Geometry: final body of the model. Coordinates: model frame, mm. Face numbers are marked on the shaded views. A direction names the side the tool comes from. Give positions to 0.01 mm unless a question says otherwise; leave off trailing zeros. Write each loop counter-clockwise with the first axis right and the second up, starting at its lowest first coordinate (ties: lowest second). Pieces come first, ordered by that corner, then holes.
Q1. Section D-D (z = 20). Return the cut outline in (x, y), plus the area to 3 significant figures.
Q2. Pin query (flat end, axial travel): pin 1 Ø1 at (x, y) = (54.5, 40.5) entering from +Z; pin 2 Ø1.9 at (x, y) = (38.5, 3.5) entering from +Z; pin 3 Ø1 at (x, y) = (32, 3.5) entering from +Z. Return the tip coordinate at first contact, or that it passes through.
Q3. Section A-A (z = 15). Return the cut outline in (x, y).
Q4. Reachability of the marked faces 1 and 2 from +Z, -Z, +X, -X, +Y, -Y: full face, straight path, thin tool, end or side. Return the list, or none.
Q5. Mould query, pull axis X, two halves, no side actions, for the marked faces 3, 4 and 5. Classes: +X half, -X half, draft (parallel to the pull), parting line (faces both ways), or undercut.
Q6. Section C-C (x = 35.5). Return the cut outline in (y, z), plus the area to 3 significant figures.
Q7. Section B-B (y = 35). Return the cut outline in (x, z).
Q8. Line query: line 1 (Y direction, x = 32, z = 23); line 2 (Y direction, x = 27, z = 22). Output: solid intervals per line, ascending.
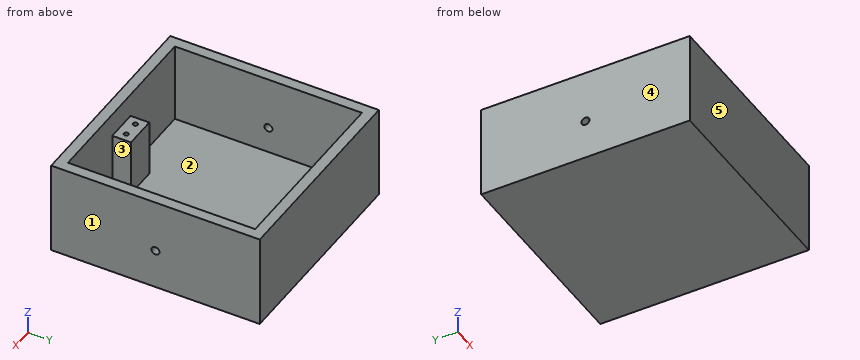
from build123d import *

# Parameters (mm, degrees)
F0_W      = 78
F0_H      = 78
F0_W_2    = 70
F0_H_2    = 70
F1_DEPTH  = 35
F2_W      = 70
F2_H      = 70
F3_DEPTH  = 5
F4_W      = 12
F4_H      = 7
F5_DEPTH  = 26.2
F7_R      = 0.85
F8_DEPTH  = 10
F10_R     = 1.5
F11_DEPTH = 25.4
F13_R     = 1.5
F14_DEPTH = 25.4


with BuildPart() as f1:
    # F0 (on Top) → F1 (new body)
    with BuildSketch(Plane.XY):
        with Locations((35, 35)):
            Rectangle(F0_W, F0_H)
        with Locations((35, 35)):
            Rectangle(F0_W_2, F0_H_2, mode=Mode.SUBTRACT)
    extrude(amount=F1_DEPTH)

    # F2 (on Top) → F3 (join)
    with BuildSketch(Plane.XY):
        with Locations((35, 35)):
            Rectangle(F2_W, F2_H)
    extrude(amount=F3_DEPTH)

    # F4 (on Top) → F5 (join)
    with BuildSketch(Plane.XY):
        with Locations((35, 3.5)):
            Rectangle(F4_W, F4_H)
    extrude(amount=F5_DEPTH)

    # F7 (on offset) → F8 (cut)
    with BuildSketch(Plane.XY.offset(26.2)):
        with Locations((38, 3.5)):
            Circle(F7_R)
        with Locations((32, 3.5)):
            Circle(F7_R)
    extrude(amount=-F8_DEPTH, mode=Mode.SUBTRACT)

    # F10 (on offset) → F11 (cut)
    with BuildSketch(Plane.YZ.offset(74)):
        with Locations((35, 15)):
            Circle(F10_R)
    extrude(amount=-F11_DEPTH, mode=Mode.SUBTRACT)

    # F13 (on offset) → F14 (cut)
    with BuildSketch(Plane(origin=(-4, 0, 0), x_dir=(0, -1, 0), z_dir=(-1, 0, 0))):
        with Locations((-35, 15)):
            Circle(F13_R)
    extrude(amount=-F14_DEPTH, mode=Mode.SUBTRACT)


solid = f1.part
Computed:
1. outline: (-4, -4) - (74, -4) - (74, 74) - (-4, 74) - close; hole (0, 0) - (29, 0) - (29, 7) - (41, 7) - (41, 0) - (70, 0) - (70, 70) - (0, 70) - close; hole circle Ø1.7 at (32, 3.5); hole circle Ø1.7 at (38, 3.5)
1. area: 1,260 mm2
2. pin 1: stops at z = 5
2. pin 2: stops at z = 26.2
2. pin 3: stops at z = 16.2
3. outline: (-4, -4) - (74, -4) - (74, 33.5) - (70, 33.5) - (70, 0) - (41, 0) - (41, 7) - (29, 7) - (29, 0) - (0, 0) - (0, 33.5) - (-4, 33.5) - close; (-4, 36.5) - (0, 36.5) - (0, 70) - (70, 70) - (70, 36.5) - (74, 36.5) - (74, 74) - (-4, 74) - close
4. face 1: +Z, -Z, +X, +Y, -Y
4. face 2: +Z
5. face 3: undercut
5. face 4: -X half
5. face 5: draft
6. outline: (-4, 0) - (74, 0) - (74, 35) - (70, 35) - (70, 5) - (7, 5) - (7, 26.2) - (0, 26.2) - (0, 35) - (-4, 35) - close
6. area: 778 mm2
7. outline: (-4, 0) - (74, 0) - (74, 13.5) - (70, 13.5) - (70, 5) - (0, 5) - (0, 13.5) - (-4, 13.5) - close; (-4, 16.5) - (0, 16.5) - (0, 35) - (-4, 35) - close; (70, 16.5) - (74, 16.5) - (74, 35) - (70, 35) - close
8. line 1: y = -4 to 2.65, 4.35 to 7, 70 to 74
8. line 2: y = -4 to 0, 70 to 74
